Source: three-view drawing plus pictorial views. Frame: mm from the lowest corner of the part. Give positions to 0.01 mm unless a question says otherwise; leave off trailing zeros. Loops run counter-clockwise (first coordinate to the right, second up) from the corner with the lowest first, then second, coordinate; pieces in that order, holes last. Notation, with made-up numbers: (74.25, 24) - (120.25, 24) arc R6 cw to (120.25, 30) - close; hole circle Ø10 at (-24, 8). An arc over 180 degrees is marked (long way). One line per item, written item: value.
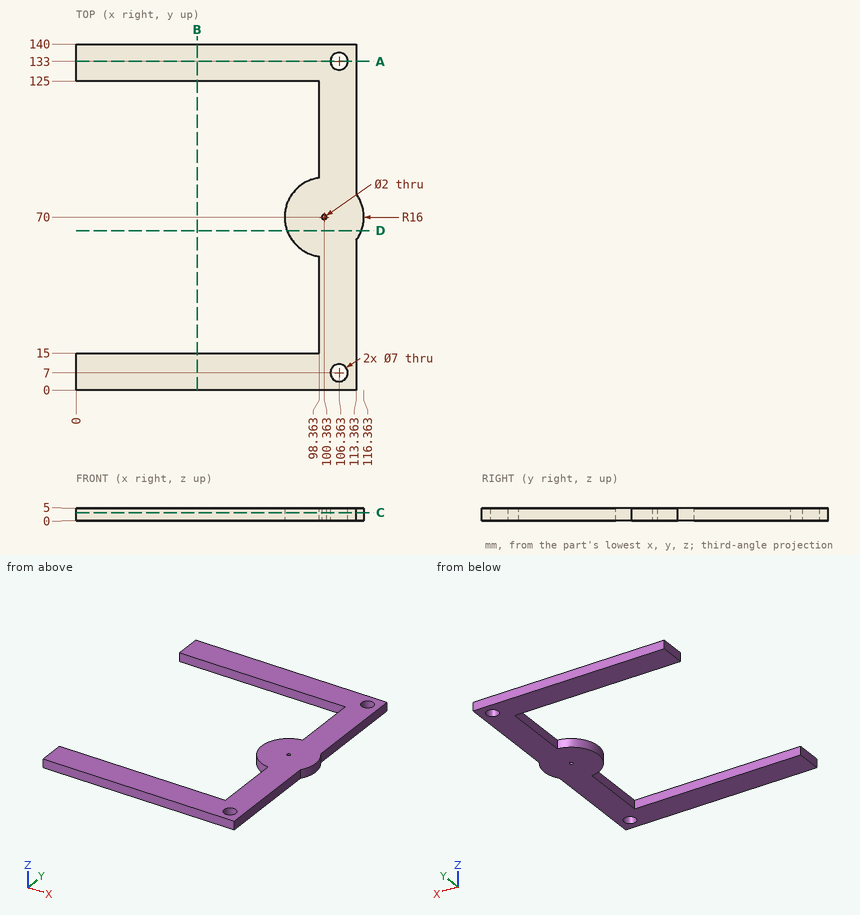
Item 1: Section A-A, the plane y = 133. Output: boundary loops of the cut face in (x, z).
Verdict:
outline: (0, 0) - (102.86, 0) - (102.86, 5) - (0, 5) - close; (109.86, 0) - (113.36, 0) - (113.36, 5) - (109.86, 5) - close
Item 2: Section C-C, the plane z = 3.2. Output: boundary loops of the cut face in (x, y), and give its area (3 significant figures).
Verdict:
outline: (0, 0) - (113.36, 0) - (113.36, 60.67) arc R16 ccw to (113.36, 79.33) - (113.36, 140) - (0, 140) - (0, 125) - (98.36, 125) - (98.36, 85.87) arc R16 ccw to (98.36, 54.13) - (98.36, 15) - (0, 15) - close; hole circle Ø2 at (100.36, 70); hole circle Ø7 at (106.36, 7); hole circle Ø7 at (106.36, 133)
area: 5,350 mm^2
Item 3: Section B-B, the plane x = 49. Output: boundary loops of the cut face in (y, z), and give its area (3 significant figures).
Verdict:
outline: (0, 0) - (15, 0) - (15, 5) - (0, 5) - close; (125, 0) - (140, 0) - (140, 5) - (125, 5) - close
area: 150 mm^2
Item 4: Pin query (flat end, axial travel): P1, Ø2.5, axis at y = 40.5, z = 3.5, coming from the -X side; P2, Ø2.5, axis at y = 39.5, z = 3, coming from the +X side; P3, Ø8, axis at x = 104, y = 64.5, coming from the -Z side. Return the tip coordinate at first contact, or that it passes through.
Verdict:
P1: stops at x = 98.36
P2: stops at x = 113.36
P3: stops at z = 0
Item 5: Material intervals for L1, parallel to Y at x = 75.5, z = 2.75; L2, parallel to Y at x = 107, z = 1.2; L3, parallel to X at y = 36.5, z = 0.2, sorted ascending.
Verdict:
L1: y = 0 to 15, 125 to 140
L2: y = 0 to 3.56, 10.44 to 129.56, 136.44 to 140
L3: x = 98.36 to 113.36
Item 6: Section D-D, the plane y = 64.5. Output: boundary loops of the cut face in (x, z), and give its area (3 significant figures).
Verdict:
outline: (85.34, 0) - (115.39, 0) - (115.39, 5) - (85.34, 5) - close
area: 150 mm^2
